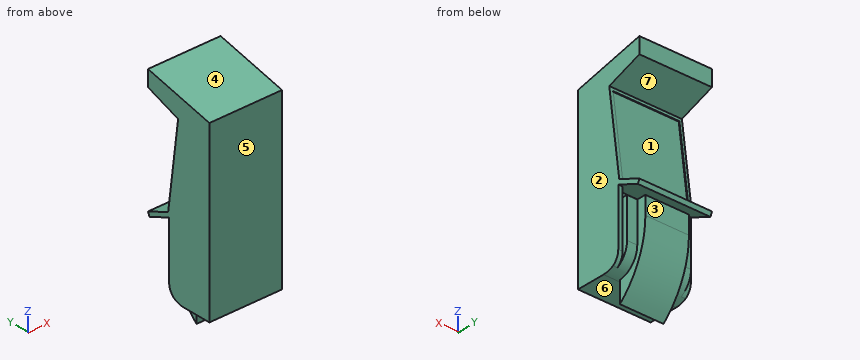
from build123d import *

# Parameters (mm, degrees)
F1_DEPTH     = 500
F2_W         = 500
F2_H         = 299.909304566
F3_DEPTH     = 213.9956919492
F4_W         = 30
F4_H         = 424.5749488473
F5_DEPTH     = 100
F6_DEPTH     = 138
F7_R         = 100
F8_W         = 70
F8_H         = 424.1601228714
F9_DEPTH     = 135
F10_F1_R     = 149.6812408671
F11_W        = 300
F11_H        = 423.4383900396
F11_H_2      = 146.1387078532
F12_DEPTH    = 198
F13_T1_DEPTH = 2527.0832943561
F14_W        = 455.9908173978
F14_H        = 558.4075003862
F15_DEPTH    = 5


# Not quite as in the source:
# - a fillet or chamfer that OpenCascade refuses, or shapes differently, is made with other operations: its cross-section is extruded or revolved along the edge and cut away or added


with BuildPart() as f1:
    # F0 (on Right) → F1 (new body)
    with BuildSketch(Plane.YZ):
        Polygon((-1006.1864304423, 680.3810487322), (-1006.1864304423, -819.6189512678), (-792.191738493, -819.6189512678), (-792.191738493, 13.2260688636), (-539.2304401761, -94.6422840199), (-527.4629834979, -67.0465060217), (-684.6932624212, 0), (-762.4113425204, 594.9452916241), (-527.4629834979, 680.3810487322), (-527.4629834979, 790.310077366), align=None)
    extrude(amount=F1_DEPTH)

    # F2 (on face) → F3 (cut, through all)
    with BuildSketch(Plane(origin=(0, -792.191738493, 0), x_dir=(-1, 0, 0), z_dir=(0, 1, 0))):
        with Locations((-250, -669.6642989848)):
            Rectangle(F2_W, F2_H)
    extrude(amount=-F3_DEPTH, mode=Mode.SUBTRACT)

    # F4 (on face) → F5 (join)
    with BuildSketch(Plane(origin=(0, -792.191738493, 0), x_dir=(-1, 0, 0), z_dir=(0, 1, 0))):
        with Locations((-15, -307.4221722782)):
            Rectangle(F4_W, F4_H)
        with Locations((-485, -307.4221722782)):
            Rectangle(F4_W, F4_H)
    extrude(amount=F5_DEPTH)

    # F6 (add): faces of the model
    f6_faces = [f1.faces().sort_by_distance(p)[0] for p in [
        (15, -742.191738493, -95.1346978545),
        (485, -742.191738493, -95.1346978545),
    ]]
    extrude(f6_faces, amount=F6_DEPTH)

    # F7
    f7_edges = [f1.edges().sort_by_distance(p)[0] for p in [
        (485, -692.191738, -519.709647),
        (15, -692.191738, -519.709647),
    ]]
    fillet(f7_edges, radius=F7_R)

    # F8 (on face) → F9 (join)
    with BuildSketch(Plane(origin=(0, -792.191738493, 0), x_dir=(-1, 0, 0), z_dir=(0, 1, 0))):
        with Locations((-435, -307.6295852661)):
            Rectangle(F8_W, F8_H)
        with Locations((-65, -307.6295852661)):
            Rectangle(F8_W, F8_H)
    extrude(amount=F9_DEPTH)

    # F10: fillet of radius 149.6812408671 on 2 edges, made by hand

    # F10_f1
    f10_f1_edges = [f1.edges().sort_by_distance(p)[0] for p in [
        (435, -657.191738493, -519.7096467018),
    ]]
    fillet(f10_f1_edges, radius=F10_F1_R)

    # F11 (on face) → F12 (join)
    with BuildSketch(Plane(origin=(0, -792.191738493, 0), x_dir=(-1, 0, 0), z_dir=(0, 1, 0))):
        with Locations((-250, -307.2687188502)):
            Rectangle(F11_W, F11_H)
        with Locations((-250, -592.0572677966)):
            Rectangle(F11_W, F11_H_2)
    extrude(amount=F12_DEPTH)

    # F13: fillet of radius 600 on 1 edges, made by hand

    # F13_s2 → F13_t1 (cut)
    with BuildSketch(Plane.YZ.offset(-1013.541647178)):
        with BuildLine():
            ThreePointArc((-792.191738493, -665.1266217232), (-645.9217320181, -463.431114991), (-594.191738493, -219.709962852))
            Line((-594.191738493, -219.709962852), (-594.191738493, -665.1266217232))
            Line((-594.191738493, -665.1266217232), (-792.191738493, -665.1266217232))
        make_face()
    extrude(amount=F13_T1_DEPTH, mode=Mode.SUBTRACT)

    # F14 (on face) → F15 (cut)
    with BuildSketch(Plane(origin=(0, -673.2054408747, -87.9412529416), x_dir=(-1, 0, 0), z_dir=(0, 0.991575486, 0.1295301335))):
        with Locations((-247.8018868715, 387.0010599494)):
            Rectangle(F14_W, F14_H)
    extrude(amount=-F15_DEPTH, mode=Mode.SUBTRACT)


solid = f1.part
Build history of the part. All positions in model axes, mm. Face numbers are marked on the shaded views. A direction names the side the tool comes from. Coordinates: 2 decimals unless noted, no trailing zeros. Write each loop counter-clockwise with the first axis right and the second up, starting at its lowest first coordinate (ties: lowest second). Pieces come first, ordered by that corner, then holes.
(1) Mould opens along Z. For the marked faces 4, 5, 6 and 7 say: pulls with the +Z half, pulls with the -Z half, needs draft (parallel to the pull), parting line crosses it, or undercut.
(2) Cut at B-B on z = -346.5. List the corners of the cut face in (x, y), and give its area (3 significant figures).
(3) Cut at D-D on x = 77. List the corners of the cut face in (y, z).
(4) Cut at A-A on x = 365. List the corners of the cut face in (y, z), and give its area (3 significant figures).
(5) Pin check, flat tips, straight feed: pin 1 Ø6 at (x, y) = (85, -904) entering from -Z; pin 2 Ø9 at (x, z) = (489, -321) entering from +Y; pin 3 Ø4 at (x, z) = (304, -341) entering from +Y. Stop position of each tip, or through.
(6) Cut at C-C on y = -608. List the corners of the cut face in (x, z).
(7) Drill centre lines: line 1 (Z direction, x = 447, y = -670); line 2 (Y direction, x = 272.5, z = -192); line 3 (Y direction, x = 182, z = 329). Where is each one in solid material? Low to high.
(8) 3-axis set-ups, long thin cutter, end or side, ignore diameter. For the marked faces 1, 2 and 3: which of +Z, -Z, +X, -X, +Y, -Y reach the whole face in a straight line?
Working result:
1. face 4: pulls with the +Z half
1. face 5: needs draft
1. face 6: pulls with the -Z half
1. face 7: undercut
2. outline: (0, -1006.19) - (500, -1006.19) - (500, -692.19) - (470, -692.19) - (470, -657.19) - (400, -657.19) - (400, -607.74) - (100, -607.74) - (100, -657.19) - (30, -657.19) - (30, -692.19) - (0, -692.19) - close
2. area: 187,000 mm2
3. outline: (-1006.19, -519.71) - (-806.87, -519.71) arc R149.68 ccw to (-657.19, -370.03) - (-657.19, -95.55) - (-792.19, -95.55) - (-792.19, 13.23) - (-539.23, -94.64) - (-527.46, -67.05) - (-684.69, 0) - (-687.17, 18.95) - (-692.13, 18.3) - (-764.46, 572) - (-759.5, 572.65) - (-762.41, 594.95) - (-527.46, 680.38) - (-527.46, 790.31) - (-1006.19, 680.38) - close
4. outline: (-1006.19, -519.71) - (-806.87, -519.71) arc R149.68 ccw to (-792.19, -518.99) - (-792.19, -665.13) arc R600 ccw to (-594.19, -219.71) - (-594.19, -95.55) - (-792.19, -95.55) - (-792.19, 13.23) - (-539.23, -94.64) - (-527.46, -67.05) - (-684.69, 0) - (-687.17, 18.95) - (-692.13, 18.3) - (-764.46, 572) - (-759.5, 572.65) - (-762.41, 594.95) - (-527.46, 680.38) - (-527.46, 790.31) - (-1006.19, 680.38) - close
4. area: 425,000 mm2
5. pin 1: stops at z = -519.71
5. pin 2: stops at y = -692.19
5. pin 3: stops at y = -606.17
6. outline: (0, -65.32) - (500, -65.32) - (500, -32.7) - (0, -32.7) - close; (0, 651.09) - (500, 651.09) - (500, 771.82) - (0, 771.82) - close; (100, -347.69) - (400, -347.69) - (400, -95.55) - (100, -95.55) - close
7. line 1: z = -430.61 to -95.55, -38.88 to -6.27, 628.55 to 757.58
7. line 2: y = -1006.19 to -594.19
7. line 3: y = -1006.19 to -732.71
8. face 1: +Y
8. face 2: +Z, -Z, +X, +Y, -Y
8. face 3: -Z, +X, -X, +Y
